For this review, take the finished solid that the model builds, in its own axes (mm). A direction names the side the tool comes from. Round coordinates to 2 decimals unless told otherwise and drop trailing zeros. Loops run counter-clockwise (first coordinate to the right, second up) from the corner with the lowest first, then second, coordinate; pieces in that order, holes last.
```python
from build123d import *

# Parameters (mm, degrees)
EXTRUDE_1_DEPTH = 10
FILLET_1_R      = 10
FILLET_2_R      = 3
SKETCH_2_R      = 3
EXTRUDE_2_DEPTH = 1
FILLET_3_R      = 0.5


with BuildPart() as part:
    # Эскиз1 → Бобышка-Вытянуть1 (new body)
    with BuildSketch(Plane.XY):
        Polygon((0, 0), (-20, -5), (0, -10), (20, -5), align=None)
    extrude(amount=EXTRUDE_1_DEPTH)

    # Скругление1
    fillet_1_edges = [part.edges().sort_by_distance(p)[0] for p in [
        (0, -10, 5),
        (0, 0, 5),
    ]]
    fillet(fillet_1_edges, radius=FILLET_1_R)

    # Скругление2
    fillet_2_edges = [part.edges().sort_by_distance(p)[0] for p in [
        (20, -5, 5),
        (-20, -5, 5),
    ]]
    fillet(fillet_2_edges, radius=FILLET_2_R)

    # Эскиз2 → Бобышка-Вытянуть2 (add)
    with BuildSketch(Plane(origin=(0, 0, 0), x_dir=(-1, 0, 0), z_dir=(0, 0, -1))):
        with Locations(Location((0, -5, 0), (0, 0, 180))):
            Circle(SKETCH_2_R)
    extrude(amount=EXTRUDE_2_DEPTH)

    # Скругление3
    fillet_3_edges = [part.edges().sort_by_distance(p)[0] for p in [
        (5.391823124, -8.652044219, 0),
        (5.391823124, -8.652044219, 10),
        (-5.391823124, -1.347955781, 0),
        (0, -0.307764064, 0),
        (0, -9.692235936, 0),
        (-5.391823124, -1.347955781, 10),
        (0, -0.307764064, 10),
        (0, -9.692235936, 10),
        (5.391823124, -1.347955781, 0),
        (5.391823124, -1.347955781, 10),
        (-5.391823124, -8.652044219, 0),
        (-10.630683123, -5, 0),
        (10.630683123, -5, 0),
        (-5.391823124, -8.652044219, 10),
        (-10.630683123, -5, 10),
        (10.630683123, -5, 10),
    ]]
    fillet(fillet_3_edges, radius=FILLET_3_R)


solid = part.part
```
(1) Insertion check: pin 1 Ø2.5 at (x, y) = (-5, -3.5) entering from -Z; pin 2 Ø1.5 at (y, z) = (-7.5, 8.5) entering from -X. Each pin has a flat end and moves straight along its axis. Give the tip position at first contact, or say it passes through.
(2) Add section B-B (x = 0). Give the boundary of the cut face in (y, z).
(3) Add section A-A (y = -5). Give the boundary of the cut face in (x, z).
(4) For faces 1 (the cylindrical face through (-5.314, -8.517, 0.143)), 2 (the cylindrical face through (-0.65, -2.07, -0.49)), list the 3-axis set-ups (+Z, -Z, +X, -X, +Y, -Y) from which the entire face can be reached by the end or side of a thin tool; tool diameter is ignored.
(5) For L1, parallel to Z at x = 0.5, y = -1.5; L2, parallel to Y at x = -0.25, z = 6.25; L3, parallel to X at y = -7.25, z = 7.75 (3 decimals), list the stretches that pass through material, from the lowest coordinate up.
Outcome:
1. pin 1: stops at z = 0
1. pin 2: stops at x = -10.07
2. outline: (-9.69, 0.5) arc R0.5 ccw to (-9.19, 0) - (-8, 0) - (-8, -1) - (-2, -1) - (-2, 0) - (-0.81, 0) arc R0.5 ccw to (-0.31, 0.5) - (-0.31, 9.5) arc R0.5 ccw to (-0.81, 10) - (-9.19, 10) arc R0.5 ccw to (-9.69, 9.5) - close
3. outline: (-10.63, 0.5) arc R0.5 ccw to (-10.13, 0) - (-3, 0) - (-3, -1) - (3, -1) - (3, 0) - (10.13, 0) arc R0.5 ccw to (10.63, 0.5) - (10.63, 9.5) arc R0.5 ccw to (10.13, 10) - (-10.13, 10) arc R0.5 ccw to (-10.63, 9.5) - close
4. face 1: -Z, -X, -Y
4. face 2: -Z
5. L1: z = 0 to 10
5. L2: y = -9.69 to -0.31
5. L3: x = -9.615 to 9.615
